Print and shaded views of the part. All mm, measured from the part's lowest x, y and z. A direction names the side the tool comes from. Give positions to 0.01 mm unless a question says otherwise; leave off trailing zeros. Loops run counter-clockwise (first coordinate to the right, second up) from the corner with the lowest first, then second, coordinate; pieces in that order, holes last. Notation, with made-up numbers: M 19.25,62 L 48.25,62 A28 cw 48.25,87 Z; hole C -26.75,60.5 d3. An arc over 180 degrees is marked long. Put each result on its own line as item: value. Start each with the question number.
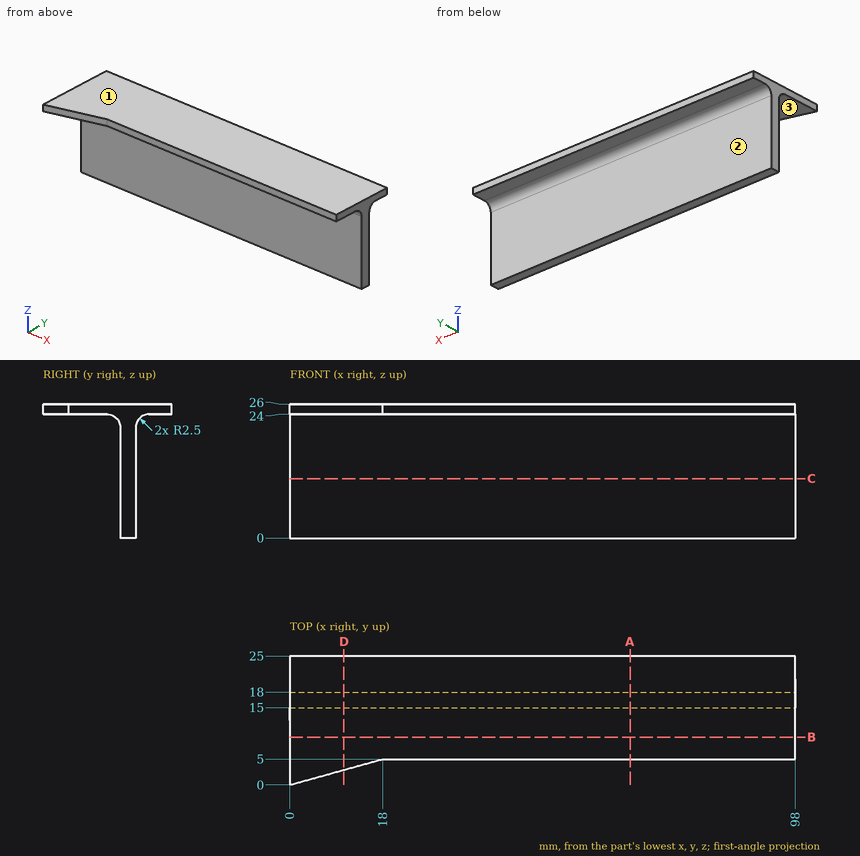
1) Band-saw the part on D-D on x = 10.5. Give the cut face in (y, z), then the cut area to 3 significant figures.
2) Band-saw the part on C-C on z = 11.5. Give the cut face in (x, y).
3) Which spindle directions (+Z, -Z, +X, -X, +Y, -Y) get a long thin tool onto all of the face, cutting with end or side? Do the marked faces 1, 2 and 3. Say none if no direction does.
4) Pin check, flat tips, straight feed: pin 1 Ø1.3 at (x, y) = (60.5, 23.5) entering from -Z; pin 2 Ø8 at (x, z) = (62, 10) entering from -Y; pin 3 Ø6 at (y, z) = (10, 5.5) entering from -X; pin 4 Ø0.6 at (x, z) = (40.5, 25.5) entering from -Y. Stop position of each tip, or through.
5) Band-saw the part on B-B on y = 9.25. Give the cut face in (x, z), then the cut area to 3 significant figures.
6) Band-saw the part on A-A on x = 66. Give the cut face in (y, z).
7) Wall check: L1, parallel to Y at x = 66, z = 17.5; L2, parallel to Z at x = 67, y = 9; L3, parallel to Y at x = 73.5, z = 24.25. Give the ranges that are in metal, low to high.
Evaluation:
1. outline: M 2.92,24 L 12.5,24 A2.5 cw 15,21.5 L 15,0 L 18,0 L 18,21.5 A2.5 cw 20.5,24 L 25,24 L 25,26 L 2.92,26 Z
1. area: 119 mm2
2. outline: M 0,15 L 98,15 L 98,18 L 0,18 Z
3. face 1: +Z, +X, -X, +Y, -Y
3. face 2: -Z, +X, -X, +Y
3. face 3: -Z, +X, -X, -Y
4. pin 1: z = 24
4. pin 2: y = 15
4. pin 3: through
4. pin 4: y = 5
5. outline: M 0,24 L 98,24 L 98,26 L 0,26 Z
5. area: 196 mm2
6. outline: M 5,24 L 12.5,24 A2.5 cw 15,21.5 L 15,0 L 18,0 L 18,21.5 A2.5 cw 20.5,24 L 25,24 L 25,26 L 5,26 Z
7. L1: 15 to 18
7. L2: 24 to 26
7. L3: 5 to 25
